Geometry check sheet. Reference: drawing and pictorial views, mm from the part's lowest x, y, z. A direction names the side the tool comes from. Round coordinates to 2 decimals unless told otherwise and drop trailing zeros. Loops run counter-clockwise (first coordinate to the right, second up) from the corner with the lowest first, then second, coordinate; pieces in that order, holes last. Notation, with made-up numbers: (20.5, -18.75) - (29.5, -18.75) arc R24 cw to (29.5, 0.25) - close; hole circle Ø4 at (-19.5, 84.5). An arc over 180 degrees is marked (long way). Return JSON: item names as keys, results as strings.
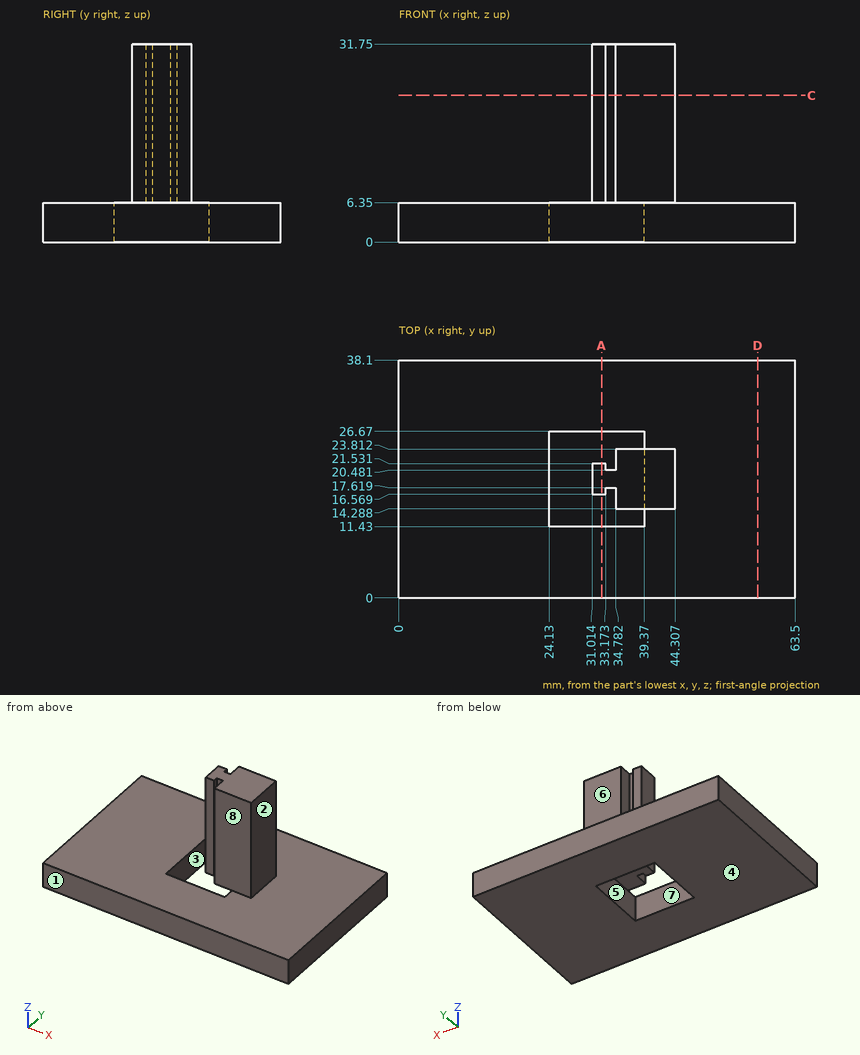
Q1. Tool access check on the marked faces 4, 5, 6, 7 and 8. Record the directions out of +Z, -Z, +X, -X, +Y, -Y that give a thin tool (end or side, any length) a straight path to the whole face; none if there is none.
Answer key:
{"face 4": "-Z, +X, -X, +Y, -Y", "face 5": "-Z", "face 6": "+Z, +X, -X, +Y", "face 7": "+Z, -Z", "face 8": "+Z, +X, -X, -Y"}
Q2. Scan lines: probe 1 along Y at (x, z) = (29, 2.5); probe 2 along X at (y, z) = (19, 2.5); probe 3 along Z at (x, y) = (52.5, 2.5). Record each from-to range of solid material in increasing order. Write a range as [from, to].
Answer key:
{"probe 1": "y = [0, 11.43], [26.67, 38.1]", "probe 2": "x = [0, 24.13], [39.37, 63.5]", "probe 3": "z = [0, 6.35]"}
Q3. Depth check by flat-ended pin: P1, Ø4, axis at y = 26.5, z = 10.5, coming from the +X side; P2, Ø2.5, axis at x = 31.5, z = 21, coming from the +Y side; P3, Ø2.5, axis at x = 34.5, y = 18, coming from the -Z side; P4, Ø5, axis at x = 40.5, z = 20, coming from the -Y side. Enter the tip coordinate at first touch or a pass-through.
Answer key:
{"P1": "passes through", "P2": "stops at y = 21.53", "P3": "stops at z = 6.35", "P4": "stops at y = 14.29"}
Q4. Sectioned sample at D-D (x = 57.5). Enter the section's corners in (y, z), plus the area to 3 significant figures.
Answer key:
{"outline": "(0, 0) - (38.1, 0) - (38.1, 6.35) - (0, 6.35) - close", "area": "242 mm²"}
Q5. Sectioned sample at C-C (z = 23.5). Enter the section's corners in (x, y) (1 decimal).
Answer key:
{"outline": "(31, 16.6) - (33.2, 16.6) - (33.2, 17.6) - (34.8, 17.6) - (34.8, 14.3) - (44.3, 14.3) - (44.3, 23.8) - (34.8, 23.8) - (34.8, 20.5) - (33.2, 20.5) - (33.2, 21.5) - (31, 21.5) - close"}
Q6. Sectioned sample at A-A (x = 32.5). Enter the section's corners in (y, z), plus the area to 3 significant figures.
Answer key:
{"outline": "(0, 0) - (11.43, 0) - (11.43, 6.35) - (0, 6.35) - close; (16.57, 6.35) - (21.53, 6.35) - (21.53, 31.75) - (16.57, 31.75) - close; (26.67, 0) - (38.1, 0) - (38.1, 6.35) - (26.67, 6.35) - close", "area": "271 mm²"}
Q7. Draft check along X on the marked faces 1, 2 and 3. Enter one of: released by +X, released by -X, zero draft, split by the parting line, or undercut.
Answer key:
{"face 1": "zero draft", "face 2": "released by +X", "face 3": "undercut"}
